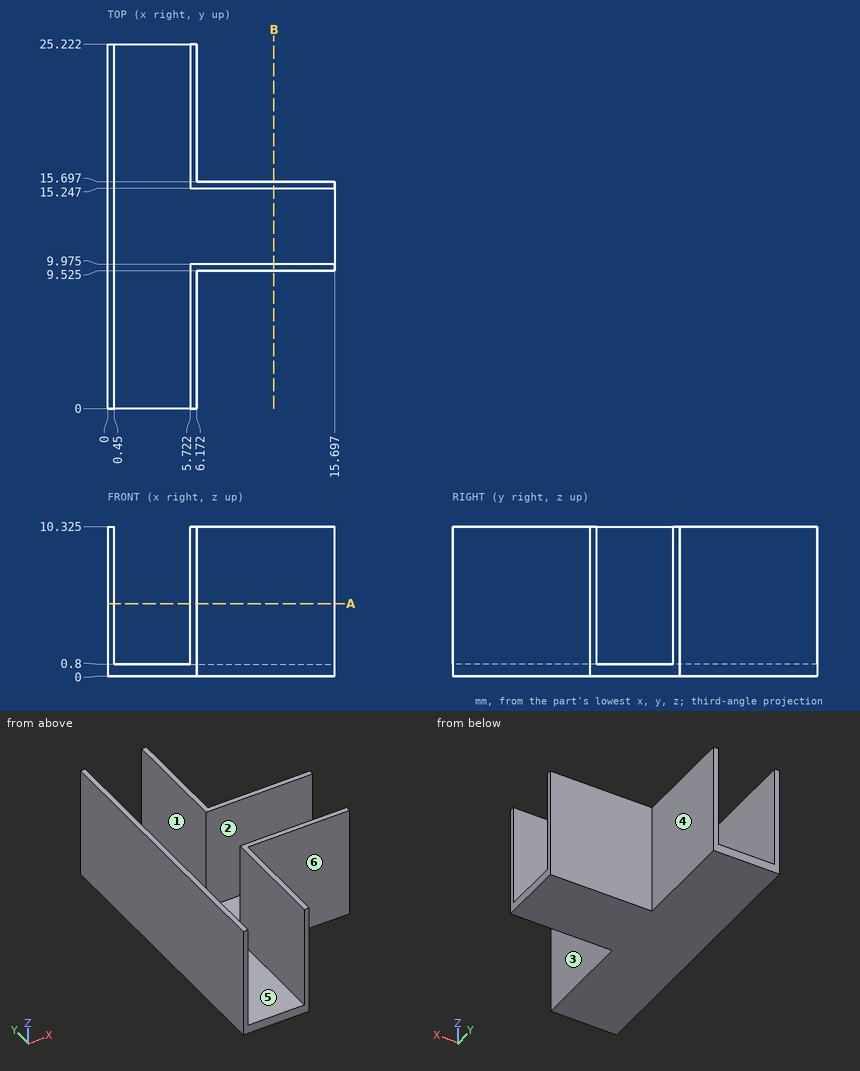
For this review, use the dimensioned drawing (mm, ordinates from the lowest corner) and the shaded views. A direction names the side the tool comes from. Give positions to 0.01 mm unless a question says otherwise; leave off trailing zeros. Order: outer loops, then holes, each group sorted by start corner. A loop starts at its lowest first (then second) coordinate and runs counter-clockwise, first axis right, second up. Notation, with made-up numbers: (80.25, -39.5) - (109.25, -39.5) arc R15 ccw to (109.25, -22.5) - close; hole circle Ø8 at (15.5, 61). An arc over 180 degrees is marked (long way). Use CSV: the item, a comma, the result in double quotes. Start each with the question number.
Q1. For line 1 (Y direction, x = 6.5, z = 6.5) (1 decimal); line 2 (X direction, y = 4, z = 5.5); line 3 (Z direction, x = 8.25, y = 11), list the stretches that pass through material, from the lowest coordinate up.
Q2. Machinability: for the marked faces 1, 2 and 3, which of the approach directions +Z, -Z, +X, -X, +Y, -Y give a long, thin tool a straight path to every point of the face, cutting with its end or side? Answer none if there is none.
Q3. Draft analysis for pull direction X (two halves, no side actions). For the marked faces 4, 5 and 6, state which applies: pulls with the +X half, pulls with the -X half, needs draft (parallel to the pull), parting line crosses it, or undercut.
Q4. For P1, Ø1.5, axis at y = 19.5, z = 7, coming from the -X side; P2, Ø3, axis at x = 9.5, z = 6.5, coming from the +Y side; P3, Ø5, axis at x = 10, z = 7, coming from the -Y side (3 decimals); P4, Ø3, axis at y = 18.5, z = 5.5, coming from the +X side, all flat-tipped, find the tip position at first contact; note any pin that passes through.
Q5. Take a section at B-B (x = 11.5). State the section outline as (y, z) points (1 decimal), and give its area (3 significant figures).
Q6. Take a section at A-A (z = 5). Count the separate pieces of the cut face and the enclosed holes in it.
Calculated:
1,line 1,"y = 9.5 to 10, 15.2 to 15.7"
1,line 2,"x = 0 to 0.45, 5.72 to 6.17"
1,line 3,"z = 0 to 0.8"
2,face 1,"+Z, +Y, -Y"
2,face 2,"+Z, +X"
2,face 3,"+Z, -Z, +X, -Y"
3,face 4,"pulls with the +X half"
3,face 5,"undercut"
3,face 6,"needs draft"
4,P1,"stops at x = 0"
4,P2,"stops at y = 15.7"
4,P3,"stops at y = 9.525"
4,P4,"stops at x = 6.17"
5,outline,"(9.5, 0) - (15.7, 0) - (15.7, 10.3) - (15.2, 10.3) - (15.2, 0.8) - (10, 0.8) - (10, 10.3) - (9.5, 10.3) - close"
5,area,"13.5 mm²"
6,separate pieces,"3"
6,enclosed holes,"0"
